Geometry: final body of the model. Coordinates: model frame, mm. Face numbers are marked on the shaded views. Coordinates: 2 decimals unless noted, no trailing zeros. Loops run counter-clockwise (first coordinate to the right, second up) from the corner with the lowest first, then second, coordinate; pieces in that order, holes last. Notation, with made-up numbers: (5.5, 44) - (22.5, 44) arc R25 ccw to (22.5, 74) - close; hole circle Ø3 at (-33.5, -29.5). An arc over 180 degrees is marked (long way). Answer in a Markdown table with one row per item.
from build123d import *

# Parameters (mm, degrees)
F0_W     = 15
F0_H     = 30
F1_DEPTH = 10
F3_DEPTH = 22
F4_R     = 0.75
F4_R_2   = 0.8
F5_DEPTH = 7
F6_R     = 3
F7_DEPTH = 8
F8_R     = 0.95
F9_DEPTH = 25.4
F10_SIZE = 0.6


with BuildPart() as f1:
    # F0 (on Top) → F1 (new body)
    with BuildSketch(Plane.XY):
        Rectangle(F0_W, F0_H)
    extrude(amount=F1_DEPTH)

    # F2 (on face) → F3 (cut)
    with BuildSketch(Plane(origin=(0, 15, 0), x_dir=(-1, 0, 0), z_dir=(0, 1, 0))):
        with BuildLine():
            ThreePointArc((-3.940234, 7.403292), (-5.06429, 3.123137), (-1.05672, 5))
            ThreePointArc((-1.05672, 5), (-1.662096, 6.609884), (-3.178234, 7.422))
            ThreePointArc((-3.178234, 7.422), (-3.559968, 7.442544), (-3.940234, 7.403292))
        make_face()
        with BuildLine():
            ThreePointArc((-3.940234, 7.403292), (-3.559968, 7.442544), (-3.178234, 7.422))
            Line((-3.178234, 7.422), (-3.178234, 10))
            Line((-3.178234, 10), (-3.940234, 10))
            Line((-3.940234, 10), (-3.940234, 7.403292))
        make_face()
    extrude(amount=-F3_DEPTH, mode=Mode.SUBTRACT)

    # F4 (on face) → F5 (cut)
    with BuildSketch(Plane.YZ.offset(7.5)):
        with Locations((13, 8.4)):
            Circle(F4_R)
        with Locations((3, 8.5)):
            Circle(F4_R_2)
    extrude(amount=-F5_DEPTH, mode=Mode.SUBTRACT)

    # F6 (on face) → F7 (cut)
    with BuildSketch(Plane.XZ.offset(15)):
        with Locations((-2.5, 5)):
            Circle(F6_R)
    extrude(amount=-F7_DEPTH, mode=Mode.SUBTRACT)

    # F8 (on face) → F9 (cut)
    with BuildSketch(Plane.XZ.offset(7)):
        with Locations((-2.5, 5)):
            Circle(F8_R)
    extrude(amount=-F9_DEPTH, mode=Mode.SUBTRACT)

    # F10
    f10_edges = [f1.edges().sort_by_distance(p)[0] for p in [
        (-3.45, 15, 5),
    ]]
    chamfer(f10_edges, length=F10_SIZE)


solid = f1.part
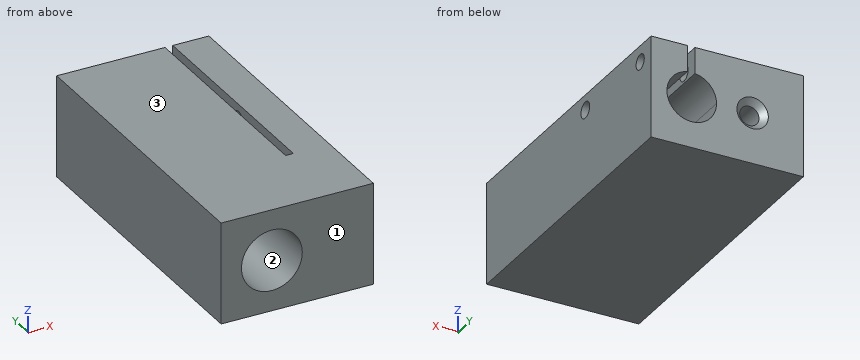
(1) Pull-direction query (Z, two-part tool) for the marked faces 1, 2 and 3; classes: pulls with the +Z half, pulls with the -Z half, needs draft (parallel to the pull), parting line crosses it, or undercut.
Verdict:
| item | result |
|---|---|
| face 1 | needs draft |
| face 2 | undercut |
| face 3 | pulls with the +Z half |
(2) Cut plane A-A on y = 3. Output: boundary loops of the cut face in (x, z).
Verdict:
| item | result |
|---|---|
| outline | (-7.5, 0) - (7.5, 0) - (7.5, 7.7) - (3.94, 7.7) - (3.94, 7.4) arc R2.44 cw (long way) to (3.18, 7.42) - (3.18, 7.7) - (0.5, 7.7) - (0.5, 9.3) - (3.18, 9.3) - (3.18, 10) - (-7.5, 10) - close; (3.94, 9.3) - (7.5, 9.3) - (7.5, 10) - (3.94, 10) - close; hole circle Ø1.9 at (-2.5, 5) |
(3) Cut plane C-C on y = 10.5. Output: boundary loops of the cut face in (x, z), then the cut area to 3 significant figures.
Verdict:
| item | result |
|---|---|
| outline | (-7.5, 0) - (7.5, 0) - (7.5, 10) - (3.94, 10) - (3.94, 7.4) arc R2.44 cw (long way) to (3.18, 7.42) - (3.18, 10) - (-7.5, 10) - close; hole circle Ø1.9 at (-2.5, 5) |
| area | 126 mm² |
(4) Ray query, probe 1 along Z at (x, y) = (2.25, 13); probe 2 along X at (y, z) = (-6.5, 4.25); probe 3 along X at (y, z) = (-3.75, 7.75). Return the intervals inside material, ascending.
Verdict:
| item | result |
|---|---|
| probe 1 | z = 0 to 2.9, 7.1 to 7.65, 9.15 to 10 |
| probe 2 | x = -7.5 to -3.08, -1.92 to 1.17, 5.83 to 7.5 |
| probe 3 | x = -7.5 to 3.18, 3.94 to 7.5 |
(5) First-contact query: pin 1 Ø1.8 at (x, z) = (-2.5, 4.5) entering from -Y; pin 2 Ø1.4 at (y, z) = (13, 8.4) entering from +X; pin 3 Ø1.5 at (x, z) = (3, 6.5) entering from +Y; pin 4 Ø1.7 at (x, z) = (-2.5, 5) entering from -Y. Flat tips, straight axial feed; report the tip coordinate or a pass-through.
Verdict:
| item | result |
|---|---|
| pin 1 | stops at y = -7 |
| pin 2 | stops at x = 0.5 |
| pin 3 | stops at y = -7 |
| pin 4 | passes through |
(6) Cut plane B-B on x = -2.5. Output: boundary loops of the cut face in (y, z), then the cut area to 3 significant figures.
Verdict:
| item | result |
|---|---|
| outline | (-15, 0) - (15, 0) - (15, 3.45) - (14.4, 4.05) - (-7, 4.05) - (-7, 2) - (-15, 2) - close; (-15, 8) - (-7, 8) - (-7, 5.95) - (14.4, 5.95) - (15, 6.55) - (15, 10) - (-15, 10) - close |
| area | 210 mm² |
(7) Cut plane D-D on x = 5.25. Output: boundary loops of the cut face in (y, z), then the cut area to 3 significant figures.
Verdict:
| item | result |
|---|---|
| outline | (-15, 0) - (15, 0) - (15, 3.29) - (-7, 3.29) - (-7, 6.71) - (15, 6.71) - (15, 10) - (-15, 10) - close; hole circle Ø1.6 at (3, 8.5); hole circle Ø1.5 at (13, 8.4) |
| area | 221 mm² |
